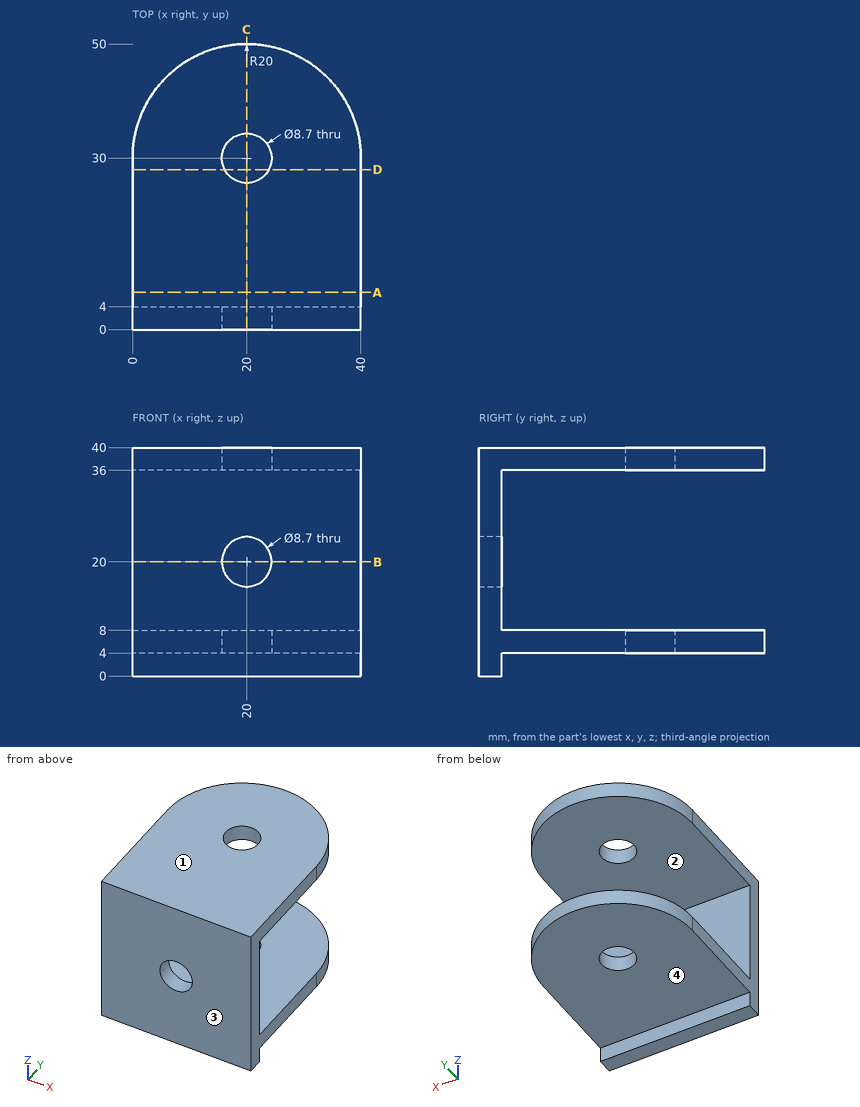
Geometry: see drawing. Coordinates: mm, zero at the bounding-box minimum. Coordinates: 2 decimals unless noted, no trailing zeros. Loops run counter-clockwise (first coordinate to the right, second up) from the corner with the lowest first, then second, coordinate; pieces in that order, holes last.
Q1. Cut plane D-D (y = 28). Output: boundary loops of the cut face in (x, z).
Q2. Cut plane C-C (x = 20). Output: boundary loops of the cut face in (y, z).
Q3. Draft query along Z for the marked faces 1, 2, 3 and 4. Return one class per face: +Z half, -Z half, draft (parallel to the pull), parting line (faces both ways), or undercut.
Q4. Contact query for flat-ended pins moving along their axis: pin 1 (12 mm diameter, centred on y = 25, z = 19, fed in from -X); pin 2 (12 mm diameter, centred on x = 17.5, y = 18.5, fed in from -Z); pin 3 (14 mm diameter, centred on x = 20, z = 26, fed in from +Y). Output: stop coordinate, or through.
Q5. Cut plane A-A (y = 6.5). Output: boundary loops of the cut face in (x, z), then the cut area to 3 significant figures.
Q6. Material intervals for line 1 (Z direction, x = 20.5, y = 42); line 2 (X direction, y = 30, z = 39); line 3 (Y direction, x = 25.5, z = 31.5), sorted ascending.
Q7. Cut plane B-B (z = 20). Output: boundary loops of the cut face in (x, y), then the cut area to 3 significant figures.
Working result:
1. outline: (0, 4) - (16.14, 4) - (16.14, 8) - (0, 8) - close; (0, 36) - (16.14, 36) - (16.14, 40) - (0, 40) - close; (23.86, 4) - (40, 4) - (40, 8) - (23.86, 8) - close; (23.86, 36) - (40, 36) - (40, 40) - (23.86, 40) - close
2. outline: (0, 0) - (4, 0) - (4, 4) - (25.65, 4) - (25.65, 8) - (4, 8) - (4, 15.65) - (0, 15.65) - close; (0, 24.35) - (4, 24.35) - (4, 36) - (25.65, 36) - (25.65, 40) - (0, 40) - close; (34.35, 4) - (50, 4) - (50, 8) - (34.35, 8) - close; (34.35, 36) - (50, 36) - (50, 40) - (34.35, 40) - close
3. face 1: +Z half
3. face 2: undercut
3. face 3: draft
3. face 4: -Z half
4. pin 1: passes through
4. pin 2: stops at z = 4
4. pin 3: stops at y = 4
5. outline: (0, 4) - (40, 4) - (40, 8) - (0, 8) - close; (0, 36) - (40, 36) - (40, 40) - (0, 40) - close
5. area: 320 mm2
6. line 1: z = 4 to 8, 36 to 40
6. line 2: x = 0 to 15.65, 24.35 to 40
6. line 3: y = 0 to 4
7. outline: (0, 0) - (15.65, 0) - (15.65, 4) - (0, 4) - close; (24.35, 0) - (40, 0) - (40, 4) - (24.35, 4) - close
7. area: 125 mm2
